```python
from build123d import *

# Parameters (mm, degrees)
PAD_DEPTH = 15


with BuildPart() as part:
    # Sketch → Pad (new body)
    with BuildSketch(Plane.XZ):
        Polygon((0, 0), (65, 0), (62.780042, -1.889917), (63.402929, -4.738076), (61.182971, -6.627993), (61.805858, -9.476152), (59.5859, -11.366069), (60.208787, -14.214228), (57.988828, -16.104145), (58.611716, -18.952304), (56.391757, -20.842221), (57.014645, -23.69038), (0, -5), align=None)
    extrude(amount=PAD_DEPTH)


solid = part.part
```
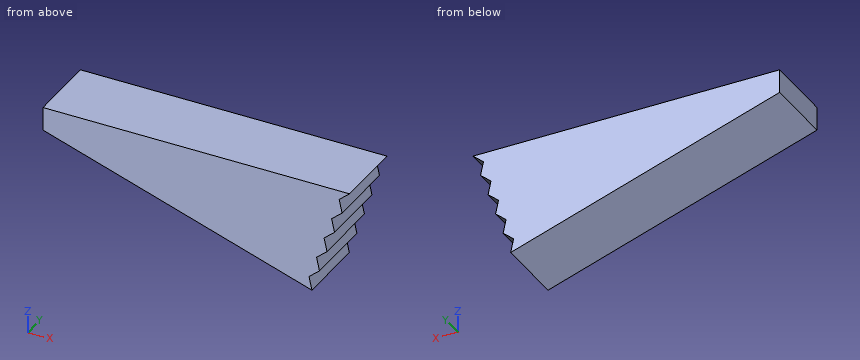
Model file for the job. Use its own axes, mm. Coordinates: 2 decimals unless noted, no trailing zeros. Write each loop counter-clockwise with the first axis right and the second up, starting at its lowest first coordinate (ties: lowest second). Pieces come first, ordered by that corner, then holes. Notation, with made-up numbers: (48.5, 3.5) - (80.5, 3.5) arc R11 ccw to (80.5, 18.5) - close; hole circle Ø9 at (-3, -36.5). An arc over 180 degrees is marked (long way). Use a Markdown table: item, result. Add a question column.
Item 1: Band-saw the part on B-B, the plane x = 42. Write the cut outline in (y, z).
Item 2: Drill centre lines: line 1 along X through (y, z) = (-6.5, -2.5); line 2 along Z through (x, y) = (30, -8.75); line 3 along Z through (x, y) = (41.5, -14). Where is each one in solid material? Low to high.
Item 3: Drop flat-ended pins along their axis: pin 1 (3 mm diameter, centred on x = 30.5, y = -2, fed in from +Z); pin 2 (6 mm diameter, centred on x = 49, y = -5, fed in from -Z); pin 3 (4 mm diameter, centred on x = 57, y = -10.5, fed in from -Z); pin 4 (5 mm diameter, centred on y = -13, z = -11, fed in from +X). Give the stop position or say it passes through.
Item 4: Band-saw the part on C-C, the plane z = -15. Write the cut outline in (x, y).
Item 5: Band-saw the part on A-A, the plane y = -3.25. Write the cut outline in (x, z), and give its area (3 significant figures).
A:
| question | item | result |
|---|---|---|
| 1 | outline | (-15, -18.77) - (0, -18.77) - (0, 0) - (-15, 0) - close |
| 2 | line 1 | x = 0 to 62.91 |
| 2 | line 2 | z = -14.83 to 0 |
| 2 | line 3 | z = -18.6 to 0 |
| 3 | pin 1 | stops at z = 0 |
| 3 | pin 2 | stops at z = -22.05 |
| 3 | pin 3 | stops at z = -23.69 |
| 3 | pin 4 | stops at x = 61.81 |
| 4 | outline | (30.5, -15) - (59.29, -15) - (59.29, 0) - (30.5, 0) - close |
| 5 | outline | (0, -5) - (57.01, -23.69) - (56.39, -20.84) - (58.61, -18.95) - (57.99, -16.1) - (60.21, -14.21) - (59.59, -11.37) - (61.81, -9.48) - (61.18, -6.63) - (63.4, -4.74) - (62.78, -1.89) - (65, 0) - (0, 0) - close |
| 5 | area | 894 mm² |
